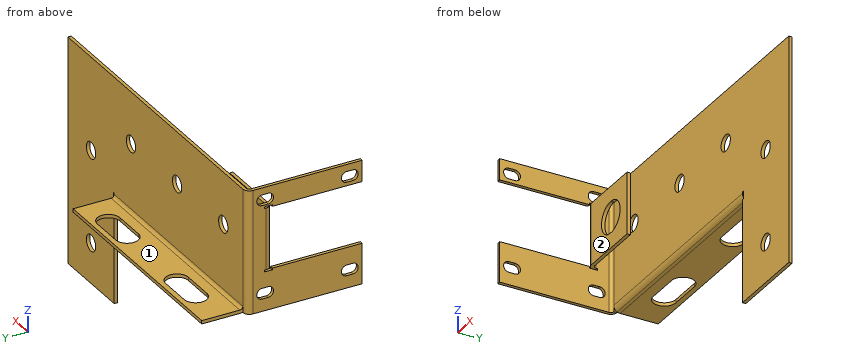
from build123d import *

# Parameters (mm, degrees)
BASE_FLANGE2_DEPTH           = 0.8128
EDGE_FLANGE1_STRIP_W         = 4.7244
EDGE_FLANGE1_STRIP_H         = 0.8128
EDGE_FLANGE1_STRIP_CUT_DEPTH = 30
EDGE_FLANGE1_DEPTH           = 30
EDGE_FLANGE1_FLAT_DEPTH      = 0.8128
EDGE_FLANGE3_START           = 0.7366
EDGE_FLANGE3_DEPTH           = 55.857
EDGE_FLANGE3_START_2         = 56.1872
EDGE_FLANGE3_2_DEPTH         = 0.4064
EDGE_FLANGE3_3_DEPTH         = 55.4506
CUT_EXTRUDE1_REACH           = 92.529
SKETCH21_R                   = 2
CUT_EXTRUDE2_REACH           = 87.061
EDGE_FLANGE4_START           = -5.5664
EDGE_FLANGE4_DEPTH           = 15.8128
EDGE_FLANGE4_2_DEPTH         = 0.4064
EDGE_FLANGE4_START_2         = 9.84
EDGE_FLANGE4_3_DEPTH         = 0.4064
EDGE_FLANGE4_START_3         = -5.16
EDGE_FLANGE4_4_DEPTH         = 15
CUT_EXTRUDE3_REACH           = 90.774
CUT_EXTRUDE4_REACH           = 91.35


# Read off the part's stored shape, not the designer's step: Edge-Flange3, Edge-Flange4
# Sheet-metal steps are written as plain solids
with BuildPart() as part:
    # Sketch7 → Base-Flange2 (new body)
    with BuildSketch(Plane.YZ):
        Polygon((-14.0628, 9.84), (7.7628, 9.84), (7.7628, -5.16), (-14.0628, -5.16), (-14.0628, -15), (14.0628, -15), (14.0628, 15), (-14.0628, 15), align=None)
    extrude(amount=-BASE_FLANGE2_DEPTH)

    # Edge-Flange1 strip (across the edge) → Edge-Flange1 strip cut (cut)
    with BuildSketch(Plane(origin=(0, 14.0628, -15), x_dir=(0, -1, 0), z_dir=(0, 0, 1))):
        with Locations((-0.8128, -0.4064)):
            Rectangle(EDGE_FLANGE1_STRIP_W, EDGE_FLANGE1_STRIP_H)
    extrude(amount=EDGE_FLANGE1_STRIP_CUT_DEPTH, mode=Mode.SUBTRACT)

    # Edge-Flange1 bend section (across the edge) → Edge-Flange1 (add)
    with BuildSketch(Plane(origin=(0, 14.0628, -15), x_dir=(0, -1, 0), z_dir=(0, 0, 1))):
        with BuildLine():
            Line((0, 0.7366), (0.8128, 0.7366))
            ThreePointArc((0.8128, 0.7366), (1.028545145, 0.215745145), (1.5494, 0))
            Line((1.5494, 0), (1.5494, -0.8128))
            ThreePointArc((1.5494, -0.8128), (0.453808753, -0.358991247), (0, 0.7366))
        make_face()
    extrude(amount=EDGE_FLANGE1_DEPTH)

    # Edge-Flange1 profile (on flange) → Edge-Flange1 flat (add)
    with BuildSketch(Plane.ZX.offset(14.0628)):
        Polygon((-40, 56.1872), (-15, 56.1872), (-15, 0.7366), (15, 0.7366), (15, 76.1872), (-40, 76.1872), align=None)
    extrude(amount=-EDGE_FLANGE1_FLAT_DEPTH)

    # Edge-Flange3 outline → Edge-Flange3 (cut)
    with BuildSketch(Plane.YZ.offset(EDGE_FLANGE3_START)):
        with BuildLine():
            Line((14.0628, -15), (14.0628, -14.813707039))
            ThreePointArc((14.0628, -14.813707039), (13.468624211, -14.244121367), (13.25, -13.4506))
            Line((13.25, -13.4506), (13.25, -15))
            Line((13.25, -15), (14.0628, -15))
        make_face()
    extrude(amount=EDGE_FLANGE3_DEPTH, mode=Mode.SUBTRACT)

    # Edge-Flange3 2 outline → Edge-Flange3 2 (cut)
    with BuildSketch(Plane.YZ.offset(EDGE_FLANGE3_START_2)):
        with BuildLine():
            ThreePointArc((13.25, -13.4506), (13.468624211, -14.244121367), (14.0628, -14.813707039))
            Line((14.0628, -14.813707039), (14.0628, -13.0442))
            Line((14.0628, -13.0442), (13.25, -13.0442))
            Line((13.25, -13.0442), (13.25, -13.4506))
        make_face()
    extrude(amount=EDGE_FLANGE3_2_DEPTH, mode=Mode.SUBTRACT)

    # Edge-Flange3 3 outline → Edge-Flange3 3 (add)
    with BuildSketch(Plane.YZ.offset(EDGE_FLANGE3_START)):
        with BuildLine():
            Line((14.7994, -15), (24.0628, -15))
            Line((24.0628, -15), (24.0628, -14.1872))
            Line((24.0628, -14.1872), (14.7994, -14.1872))
            ThreePointArc((14.7994, -14.1872), (14.278545145, -13.971454855), (14.0628, -13.4506))
            Line((14.0628, -13.4506), (14.0628, -14.813707039))
            ThreePointArc((14.0628, -14.813707039), (14.419503755, -14.952704924), (14.7994, -15))
        make_face()
    extrude(amount=EDGE_FLANGE3_3_DEPTH)

    # Sketch21 → Cut-Extrude1 (cut, up to next)
    with BuildSketch(Plane(origin=(0, 14.0628, 0), x_dir=(-1, 0, 0), z_dir=(0, 1, 0)), mode=Mode.PRIVATE) as cut_extrude1_sk1:
        with Locations((-66.1872, -30.16)):
            Circle(SKETCH21_R)
    cut_extrude1_tool1 = extrude(cut_extrude1_sk1.sketch, amount=-CUT_EXTRUDE1_REACH, mode=Mode.PRIVATE) & part.part
    # Sketch21 → Cut-Extrude1 (cut, up to next)
    with BuildSketch(Plane(origin=(0, 14.0628, 0), x_dir=(-1, 0, 0), z_dir=(0, 1, 0)), mode=Mode.PRIVATE) as cut_extrude1_sk2:
        with Locations((-66.1872, -7.66)):
            Circle(SKETCH21_R)
    cut_extrude1_tool2 = extrude(cut_extrude1_sk2.sketch, amount=-CUT_EXTRUDE1_REACH, mode=Mode.PRIVATE) & part.part
    # Sketch21 → Cut-Extrude1 (cut, up to next)
    with BuildSketch(Plane(origin=(0, 14.0628, 0), x_dir=(-1, 0, 0), z_dir=(0, 1, 0)), mode=Mode.PRIVATE) as cut_extrude1_sk3:
        with Locations((-48.982258849, 2.34)):
            Circle(SKETCH21_R)
    cut_extrude1_tool3 = extrude(cut_extrude1_sk3.sketch, amount=-CUT_EXTRUDE1_REACH, mode=Mode.PRIVATE) & part.part
    # Sketch21 → Cut-Extrude1 (cut, up to next)
    with BuildSketch(Plane(origin=(0, 14.0628, 0), x_dir=(-1, 0, 0), z_dir=(0, 1, 0)), mode=Mode.PRIVATE) as cut_extrude1_sk4:
        with Locations((-29.082258849, 2.34)):
            Circle(SKETCH21_R)
    cut_extrude1_tool4 = extrude(cut_extrude1_sk4.sketch, amount=-CUT_EXTRUDE1_REACH, mode=Mode.PRIVATE) & part.part
    # Sketch21 → Cut-Extrude1 (cut, up to next)
    with BuildSketch(Plane(origin=(0, 14.0628, 0), x_dir=(-1, 0, 0), z_dir=(0, 1, 0)), mode=Mode.PRIVATE) as cut_extrude1_sk5:
        with Locations((-9.182258849, 2.34)):
            Circle(SKETCH21_R)
    cut_extrude1_tool5 = extrude(cut_extrude1_sk5.sketch, amount=-CUT_EXTRUDE1_REACH, mode=Mode.PRIVATE) & part.part
    add(cut_extrude1_tool1.solids().sort_by_distance((66.1872, 14.0628, -30.16))[0], mode=Mode.SUBTRACT)
    add(cut_extrude1_tool2.solids().sort_by_distance((66.1872, 14.0628, -7.66))[0], mode=Mode.SUBTRACT)
    add(cut_extrude1_tool3.solids().sort_by_distance((48.982259, 14.0628, 2.34))[0], mode=Mode.SUBTRACT)
    add(cut_extrude1_tool4.solids().sort_by_distance((29.082259, 14.0628, 2.34))[0], mode=Mode.SUBTRACT)
    add(cut_extrude1_tool5.solids().sort_by_distance((9.182259, 14.0628, 2.34))[0], mode=Mode.SUBTRACT)

    # Sketch22 → Cut-Extrude2 (cut, up to next)
    with BuildSketch(Plane.XY.offset(-14.1872), mode=Mode.PRIVATE) as cut_extrude2_sk1:
        with BuildLine():
            Line((10.4866, 22.8128), (18.4866, 22.8128))
            ThreePointArc((18.4866, 22.8128), (21.2366, 20.0628), (18.4866, 17.3128))
            Line((18.4866, 17.3128), (10.4866, 17.3128))
            ThreePointArc((10.4866, 17.3128), (7.7366, 20.0628), (10.4866, 22.8128))
        make_face()
    cut_extrude2_tool1 = extrude(cut_extrude2_sk1.sketch, amount=-CUT_EXTRUDE2_REACH, mode=Mode.PRIVATE) & part.part
    # Sketch22 → Cut-Extrude2 (cut, up to next)
    with BuildSketch(Plane.XY.offset(-14.1872), mode=Mode.PRIVATE) as cut_extrude2_sk2:
        with BuildLine():
            Line((47.9866, 22.8128), (39.9866, 22.8128))
            ThreePointArc((39.9866, 22.8128), (37.2366, 20.0628), (39.9866, 17.3128))
            Line((39.9866, 17.3128), (47.9866, 17.3128))
            ThreePointArc((47.9866, 17.3128), (50.7366, 20.0628), (47.9866, 22.8128))
        make_face()
    cut_extrude2_tool2 = extrude(cut_extrude2_sk2.sketch, amount=-CUT_EXTRUDE2_REACH, mode=Mode.PRIVATE) & part.part
    add(cut_extrude2_tool1.solids().sort_by_distance((14.4866, 20.0628, -14.1872))[0], mode=Mode.SUBTRACT)
    add(cut_extrude2_tool2.solids().sort_by_distance((43.9866, 20.0628, -14.1872))[0], mode=Mode.SUBTRACT)

    # Edge-Flange4 outline → Edge-Flange4 (cut)
    with BuildSketch(Plane.XY.offset(EDGE_FLANGE4_START)):
        with BuildLine():
            ThreePointArc((0, 7.949092961), (-0.594175789, 8.518678633), (-0.8128, 9.3122))
            Line((-0.8128, 9.3122), (-0.8128, 7.7628))
            Line((-0.8128, 7.7628), (0, 7.7628))
            Line((0, 7.7628), (0, 7.949092961))
        make_face()
    extrude(amount=EDGE_FLANGE4_DEPTH, mode=Mode.SUBTRACT)

    # Edge-Flange4 2 outline → Edge-Flange4 2 (cut)
    with BuildSketch(Plane.XY.offset(EDGE_FLANGE4_START)):
        with BuildLine():
            Line((0, 9.7186), (-0.8128, 9.7186))
            Line((-0.8128, 9.7186), (-0.8128, 9.3122))
            ThreePointArc((-0.8128, 9.3122), (-0.594175789, 8.518678633), (0, 7.949092961))
            Line((0, 7.949092961), (0, 9.7186))
        make_face()
    extrude(amount=EDGE_FLANGE4_2_DEPTH, mode=Mode.SUBTRACT)

    # Edge-Flange4 3 outline → Edge-Flange4 3 (cut)
    with BuildSketch(Plane.XY.offset(EDGE_FLANGE4_START_2)):
        with BuildLine():
            Line((0, 9.7186), (-0.8128, 9.7186))
            Line((-0.8128, 9.7186), (-0.8128, 9.3122))
            ThreePointArc((-0.8128, 9.3122), (-0.594175789, 8.518678633), (0, 7.949092961))
            Line((0, 7.949092961), (0, 9.7186))
        make_face()
    extrude(amount=EDGE_FLANGE4_3_DEPTH, mode=Mode.SUBTRACT)

    # Edge-Flange4 4 outline → Edge-Flange4 4 (add)
    with BuildSketch(Plane.XY.offset(EDGE_FLANGE4_START_3)):
        with BuildLine():
            ThreePointArc((0.7366, 8.5756), (0.215745145, 8.791345145), (0, 9.3122))
            Line((0, 9.3122), (0, 7.949092961))
            ThreePointArc((0, 7.949092961), (0.356703755, 7.810095076), (0.7366, 7.7628))
            Line((0.7366, 7.7628), (16.1872, 7.7628))
            Line((16.1872, 7.7628), (16.1872, 8.5756))
            Line((16.1872, 8.5756), (0.7366, 8.5756))
        make_face()
    extrude(amount=EDGE_FLANGE4_4_DEPTH)

    # Sketch27 → Cut-Extrude3 (cut, up to next)
    with BuildSketch(Plane.XZ.offset(-7.7628), mode=Mode.PRIVATE) as cut_extrude3_sk1:
        with BuildLine():
            Line((9.382258849, -1.46), (8.982258849, -1.46))
            ThreePointArc((8.982258849, -1.46), (5.182258849, 2.34), (8.982258849, 6.14))
            Line((8.982258849, 6.14), (9.382258849, 6.14))
            ThreePointArc((9.382258849, 6.14), (13.182258849, 2.34), (9.382258849, -1.46))
        make_face()
    cut_extrude3_tool1 = extrude(cut_extrude3_sk1.sketch, amount=-CUT_EXTRUDE3_REACH, mode=Mode.PRIVATE) & part.part
    add(cut_extrude3_tool1.solids().sort_by_distance((9.182259, 7.7628, 2.34))[0], mode=Mode.SUBTRACT)

    # Sketch33 → Cut-Extrude4 (cut, up to next)
    with BuildSketch(Plane.YZ, mode=Mode.PRIVATE) as cut_extrude4_sk1:
        with BuildLine():
            Line((-11.8128, 13.3), (-10.3128, 13.3))
            ThreePointArc((-10.3128, 13.3), (-9.0128, 12), (-10.3128, 10.7))
            Line((-10.3128, 10.7), (-11.8128, 10.7))
            ThreePointArc((-11.8128, 10.7), (-13.1128, 12), (-11.8128, 13.3))
        make_face()
    cut_extrude4_tool1 = extrude(cut_extrude4_sk1.sketch, amount=-CUT_EXTRUDE4_REACH, mode=Mode.PRIVATE) & part.part
    # Sketch33 → Cut-Extrude4 (cut, up to next)
    with BuildSketch(Plane.YZ, mode=Mode.PRIVATE) as cut_extrude4_sk2:
        with BuildLine():
            Line((8.7634, 10.7), (10.2634, 10.7))
            ThreePointArc((10.2634, 10.7), (11.5634, 12), (10.2634, 13.3))
            Line((10.2634, 13.3), (8.7634, 13.3))
            ThreePointArc((8.7634, 13.3), (7.4634, 12), (8.7634, 10.7))
        make_face()
    cut_extrude4_tool2 = extrude(cut_extrude4_sk2.sketch, amount=-CUT_EXTRUDE4_REACH, mode=Mode.PRIVATE) & part.part
    # Sketch33 → Cut-Extrude4 (cut, up to next)
    with BuildSketch(Plane.YZ, mode=Mode.PRIVATE) as cut_extrude4_sk3:
        with BuildLine():
            Line((8.7634, -12), (10.2634, -12))
            ThreePointArc((10.2634, -12), (11.5634, -10.7), (10.2634, -9.4))
            Line((10.2634, -9.4), (8.7634, -9.4))
            ThreePointArc((8.7634, -9.4), (7.4634, -10.7), (8.7634, -12))
        make_face()
    cut_extrude4_tool3 = extrude(cut_extrude4_sk3.sketch, amount=-CUT_EXTRUDE4_REACH, mode=Mode.PRIVATE) & part.part
    # Sketch33 → Cut-Extrude4 (cut, up to next)
    with BuildSketch(Plane.YZ, mode=Mode.PRIVATE) as cut_extrude4_sk4:
        with BuildLine():
            Line((-11.8128, -12), (-10.3128, -12))
            ThreePointArc((-10.3128, -12), (-9.0128, -10.7), (-10.3128, -9.4))
            Line((-10.3128, -9.4), (-11.8128, -9.4))
            ThreePointArc((-11.8128, -9.4), (-13.1128, -10.7), (-11.8128, -12))
        make_face()
    cut_extrude4_tool4 = extrude(cut_extrude4_sk4.sketch, amount=-CUT_EXTRUDE4_REACH, mode=Mode.PRIVATE) & part.part
    add(cut_extrude4_tool1.solids().sort_by_distance((0, -11.0628, 12))[0], mode=Mode.SUBTRACT)
    add(cut_extrude4_tool2.solids().sort_by_distance((0, 9.5134, 12))[0], mode=Mode.SUBTRACT)
    add(cut_extrude4_tool3.solids().sort_by_distance((0, 9.5134, -10.7))[0], mode=Mode.SUBTRACT)
    add(cut_extrude4_tool4.solids().sort_by_distance((0, -11.0628, -10.7))[0], mode=Mode.SUBTRACT)


solid = part.part
The listing builds one solid part. Answer for the finished solid, in the listing's coordinates (mm). Face numbers are marked on the shaded views. A direction names the side the tool comes from. Coordinates: 2 decimals unless noted, no trailing zeros. Loops run counter-clockwise (first coordinate to the right, second up) from the corner with the lowest first, then second, coordinate; pieces in that order, holes last. Notation, with made-up numbers: (-33, 73) -> (-16, 73) arc R14 ccw to (-16, 88) -> close; hole circle Ø4 at (14, -30). An arc over 180 degrees is marked (long way). Write item = value, one per line. Start each with the question number.
1) Straight lines are drawn through the part: line 1 (Y direction, x = 53, z = 0.5); line 2 (Z direction, x = 24, y = 16); line 3 (X direction, y = 13.5, z = -17.5). For each, find the intervals that lie inside material, in ascending order. Write a range as from..to.
2) A tool of negligible diameter and unlimited length cuts with its end or side. For the marked faces 1 and 2, from which of +Z, -Z, +X, -X, +Y, -Y can it reach the whole face along a straight path? Write none if from no direction.
3) A cutting plane is placed at A-A (z = -10.7). Give the vertices of the cut face in (x, y), then the cut area to 3 significant figures.
4) A cutting plane is placed at B-B (y = 2). Give the vertices of the cut face in (x, z).
5) Given pin 1 Ø4.5 at (x, y) = (20, 17.5) entering from +Z; pin 2 Ø0.9 at (x, y) = (-0.5, -4.5) entering from -Z; pin 3 Ø3 at (x, z) = (40.5, -11) entering from +Y, each flat-ended and moving along its own axis, determine where each tip first touches the part or whether it passes through.
6) A cutting plane is placed at D-D (x = 49.5). Give the vertices of the cut face in (y, z).
7) A cutting plane is placed at C-C (z = -30.16). Give the vertices of the cut face in (x, y), then the cut area to 3 significant figures.
Responses:
q1.line_1 = 13.25..14.06
q1.line_2 = -15..-14.19
q1.line_3 = 56.19..76.19
q2.face_1 = +Z, +X, -X, +Y
q2.face_2 = +Z, -Z, +X, -X, -Y
q3.outline = (-0.81, -14.06) -> (0, -14.06) -> (0, -13.11) -> (-0.81, -13.11) -> close; (-0.81, -9.01) -> (0, -9.01) -> (0, 7.46) -> (-0.81, 7.46) -> close; (-0.81, 11.56) -> (0, 11.56) -> (0, 12.51) arc R0.74 cw to (0.74, 13.25) -> (76.19, 13.25) -> (76.19, 14.06) -> (0.74, 14.06) arc R1.55 ccw to (-0.81, 12.51) -> close
q3.area = 77.7 mm²
q4.outline = (-0.81, -15) -> (0, -15) -> (0, -5.16) -> (-0.81, -5.16) -> close; (-0.81, 9.84) -> (0, 9.84) -> (0, 15) -> (-0.81, 15) -> close
q5.pin_1 = -14.19
q5.pin_2 = -15
q5.pin_3 = 14.06
q6.outline = (13.25, -13.45) arc R1.55 ccw to (14.8, -15) -> (17.77, -15) -> (17.77, -14.19) -> (14.8, -14.19) arc R0.74 cw to (14.06, -13.45) -> (14.06, 0.41) -> (13.25, 0.41) -> close; (13.25, 4.27) -> (14.06, 4.27) -> (14.06, 15) -> (13.25, 15) -> close; (22.36, -15) -> (24.06, -15) -> (24.06, -14.19) -> (22.36, -14.19) -> close
q7.outline = (56.19, 13.25) -> (64.19, 13.25) -> (64.19, 14.06) -> (56.19, 14.06) -> close; (68.19, 13.25) -> (76.19, 13.25) -> (76.19, 14.06) -> (68.19, 14.06) -> close
q7.area = 13.0 mm²
